Verification items for the finished model (mm, model axes). A direction names the side the tool comes from. Round coordinates to 2 decimals unless told otherwise and drop trailing zeros. Answer as a JSON object with one key per item and string values.
```python
from build123d import *

# Parameters (mm, degrees)
BOSS_EXTRUDE1_DEPTH     = 103
FILLET1_R               = 0.0001
SKETCH2_W               = 130
SKETCH2_H               = 105
BOSS_EXTRUDE2_DEPTH     = 10.6
FILLET2_R               = 5
SKETCH3_W               = 130
SKETCH3_H               = 105
BOSS_EXTRUDE3_DEPTH     = 16
FILLET3_R               = 5
CUT_EXTRUDE1_DEPTH      = 539.168188348
CUT_EXTRUDE1_DEPTH_BACK = 104
SKETCH4_R               = 15
SKETCH5_R               = 15
CUT_EXTRUDE2_DEPTH      = 104


with BuildPart() as part:
    # Sketch1 → Boss-Extrude1 (new body)
    with BuildSketch(Plane(origin=(0, 0, 0), x_dir=(1, 0, 0), z_dir=(0, 1, 0))):
        Polygon((0, -89.5), (0, 89.5), (517.159308144, 60), (517.159308144, -60), align=None)
    extrude(amount=BOSS_EXTRUDE1_DEPTH)

    # Fillet1
    fillet1_edges = [part.edges().sort_by_distance(p)[0] for p in [
        (0, 0, 0),
        (0, 51.5, -89.5),
        (258.579654072, 0, -74.75),
        (517.159308144, 51.5, -60),
        (517.159308144, 0, 0),
        (517.159308144, 51.5, 60),
        (258.579654072, 0, 74.75),
        (0, 51.5, 89.5),
        (0, 103, 0),
        (517.159308144, 103, 0),
        (258.579654072, 103, -74.75),
        (258.579654072, 103, 74.75),
    ]]
    fillet(fillet1_edges, radius=FILLET1_R)

    # Sketch2 → Boss-Extrude2 (add)
    with BuildSketch(Plane(origin=(0, 103, 0), x_dir=(1, 0, 0), z_dir=(0, 1, 0))):
        with Locations((437.159208144, 4.349038924)):
            Rectangle(SKETCH2_W, SKETCH2_H)
    extrude(amount=BOSS_EXTRUDE2_DEPTH)

    # Fillet2
    fillet2_edges = [part.edges().sort_by_distance(p)[0] for p in [
        (502.159208144, 108.3, 48.150961076),
        (502.159208144, 108.3, -56.849038924),
        (372.159208144, 108.3, -56.849038924),
        (372.159208144, 108.3, 48.150961076),
        (502.159208144, 113.6, -4.349038924),
        (437.159208144, 113.6, -56.849038924),
        (372.159208144, 113.6, -4.349038924),
        (437.159208144, 113.6, 48.150961076),
    ]]
    fillet(fillet2_edges, radius=FILLET2_R)

    # Sketch3 → Boss-Extrude3 (add)
    with BuildSketch(Plane(origin=(0, 103, 0), x_dir=(1, 0, 0), z_dir=(0, 1, 0))):
        with Locations((215.0001, 0)):
            Rectangle(SKETCH3_W, SKETCH3_H)
    extrude(amount=BOSS_EXTRUDE3_DEPTH)

    # Fillet3
    fillet3_edges = [part.edges().sort_by_distance(p)[0] for p in [
        (280.0001, 111, 52.5),
        (280.0001, 111, -52.5),
        (150.0001, 111, -52.5),
        (150.0001, 111, 52.5),
        (280.0001, 119, 0),
        (215.0001, 119, -52.5),
        (150.0001, 119, 0),
        (215.0001, 119, 52.5),
    ]]
    fillet(fillet3_edges, radius=FILLET3_R)

    # Sketch4 → Cut-Extrude1 (cut, two sides: drawn at the far end of the back side and taken through both)
    with BuildSketch(Plane.XZ.offset(-CUT_EXTRUDE1_DEPTH_BACK)):
        with Locations(Location((479.159308144, 0, 0), (0, 0, 90))):
            Circle(SKETCH4_R)
    extrude(amount=CUT_EXTRUDE1_DEPTH + CUT_EXTRUDE1_DEPTH_BACK, mode=Mode.SUBTRACT)

    # Sketch5 → Cut-Extrude2 (cut)
    with BuildSketch(Plane.XZ):
        with Locations(Location((255, 0, 0), (0, 0, 270))):
            Circle(SKETCH5_R)
    extrude(amount=-CUT_EXTRUDE2_DEPTH, mode=Mode.SUBTRACT)


solid = part.part
```
Q1. Set-up check for faces 1 (the flat face through (214, 119, -1)), 2 (the flat face through (280, 108, 1)), 3 (the flat face through (436, 113.6, -5)), 4 (the flat face through (150, 108, 1)), 5 (the cylindrical face through (269.872, 51.272, 1.953)): record each of +Z, -Z, +X, -X, +Y, -Y from which the full face is reachable in a straight line by a thin tool's end or side.
Geometry check:
{"face 1": "+Z, -Z, +X, -X, +Y", "face 2": "+Z, -Z, +Y", "face 3": "+Z, -Z, +X, +Y", "face 4": "+Z, -Z, -X, +Y", "face 5": "-Y"}
Q2. Release check for a two-part mould opening along X. For faces 6 (the flat face through (262.2, 50.779, 74.543)), 7 (the flat face through (479, 104, 0)), 8 (the flat face through (214, 108, 52.5)) record: released by +X, released by -X, zero draft, split by the parting line, or undercut.
Geometry check:
{"face 6": "released by +X", "face 7": "undercut", "face 8": "zero draft"}
Q3. Material ranges on line 1 along X through (y, z) = (73, 0); line 2 along Y through (x, z) = (444.5, 26.5); line 3 along Y through (x, z) = (72, 27.5), recorded low to high. Write a range as [from, to].
Geometry check:
{"line 1": "x = [0, 240], [270, 464.16], [494.16, 517.16]", "line 2": "y = [0, 113.6]", "line 3": "y = [0, 103]"}
Q4. Section check B-B, the plane y = 39. State how many separate pieces and enclosed holes the cut face has, then the cut area to 3 significant figures.
Geometry check:
{"separate pieces": "1", "enclosed holes": "2", "area": "75,900 mm2"}
Q5. Gauge pin test, flat ends, axial feed: P1, Ø10, axis at x = 241, y = 79, coming from the +Z side; P2, Ø9, axis at y = 109.5, z = -3, coming from the +X side; P3, Ø4, axis at x = 56, y = 15.5, coming from the -Z side. Record the tip position at first contact, or that the pin passes through.
Geometry check:
{"P1": "stops at z = 76.04", "P2": "stops at x = 502.16", "P3": "stops at z = -86.42"}
